Input: part model. Units: mm. Frame: model coordinates. A direction names the side the tool comes from. Give positions to 0.01 mm unless a question says otherwise; leave off trailing zeros. Order: outer loops, then holes, each group sorted by start corner. A loop starts at its lowest first (then second) coordinate and runs counter-clockwise, first axis right, second up.
```python
from build123d import *

# Parameters (mm, degrees)
BOSS_EXTRUDE1_DEPTH                 = 3.175
SKETCH2_R                           = 1.7145
SKETCH2_W                           = 20.586
SKETCH2_H                           = 41.275
CUT_FOR_MOTOR_DEPTH                 = 4.175
SKETCH3_R                           = 3.048
CUT_FOR_AXLE_DEPTH                  = 4.175
SKETCH4_W                           = 6.35
SKETCH4_H                           = 3.2258
CUT_FOR_TABS_DEPTH                  = 4.175
CUT_EXTRUDE6_DEPTH                  = 4.175
SKETCH9_W                           = 3.2258
SKETCH9_H                           = 6.35
TABS_FOR_BACK_PLATE_DEPTH           = 3.175
SKETCH10_R                          = 1.5875
CUT_FOR_BASIC_TILT_LOCK_SCREW_DEPTH = 4.175


with BuildPart() as part:
    # Sketch1 → Boss-Extrude1 (new body)
    with BuildSketch(Plane(origin=(0, 0, 0), x_dir=(0, 0, -1), z_dir=(1, 0, 0))):
        with BuildLine():
            Line((-8.901335672, 27.917328656), (29.198664328, 27.917328656))
            Line((29.198664328, 27.917328656), (52.058664328, 27.917328656))
            ThreePointArc((52.058664328, 27.917328656), (54.100437174, 20.297328656), (52.058664328, 12.677328656))
            Line((52.058664328, 12.677328656), (29.198664328, -0.520898498))
            Line((29.198664328, -0.520898498), (29.198664328, -54.632671344))
            Line((29.198664328, -54.632671344), (-8.901335672, -54.632671344))
            Line((-8.901335672, -54.632671344), (-8.901335672, 27.917328656))
        make_face()
    extrude(amount=BOSS_EXTRUDE1_DEPTH)

    # Sketch2 → cut for motor (cut, through all)
    with BuildSketch(Plane(origin=(3.175, 0, 0), x_dir=(0, 0, -1), z_dir=(1, 0, 0))):
        with Locations((12.696664328, 13.439328656)):
            Circle(SKETCH2_R)
        with Locations((2.786664328, 13.439328656)):
            Circle(SKETCH2_R)
        with Locations((12.595457687, -37.487671344)):
            Circle(SKETCH2_R)
        with Locations((2.685457687, -37.487671344)):
            Circle(SKETCH2_R)
        with Locations((7.741664328, -12.024171344)):
            Rectangle(SKETCH2_W, SKETCH2_H)
    extrude(amount=-CUT_FOR_MOTOR_DEPTH, mode=Mode.SUBTRACT)

    # Sketch3 → cut for axle (cut, through all)
    with BuildSketch(Plane(origin=(3.175, 0, 0), x_dir=(0, 0, -1), z_dir=(1, 0, 0))):
        with Locations((46.978664328, 20.297328656)):
            Circle(SKETCH3_R)
    extrude(amount=-CUT_FOR_AXLE_DEPTH, mode=Mode.SUBTRACT)

    # Sketch4 → cut for tabs (cut, through all)
    with BuildSketch(Plane(origin=(3.175, 0, 0), x_dir=(0, 0, -1), z_dir=(1, 0, 0))):
        with Locations((0.623664328, -49.920971344)):
            Rectangle(SKETCH4_W, SKETCH4_H)
        with Locations((19.673664328, -49.920971344)):
            Rectangle(SKETCH4_W, SKETCH4_H)
        Polygon((10.148664328, -54.632671344), (13.323664328, -54.632671344), (13.323664328, -51.457671344), (6.973664328, -51.457671344), (6.973664328, -54.632671344), align=None)
    extrude(amount=-CUT_FOR_TABS_DEPTH, mode=Mode.SUBTRACT)

    # Sketch8 → Cut-Extrude6 (cut, through all)
    with BuildSketch(Plane(origin=(3.175, 0, 0), x_dir=(0, 0, -1), z_dir=(1, 0, 0))):
        Polygon((29.198664328, 27.917328656), (-8.901335672, 15.979328656), (-8.901335672, 27.917328656), align=None)
    extrude(amount=-CUT_EXTRUDE6_DEPTH, mode=Mode.SUBTRACT)

    # Sketch9 → tabs for back plate (add)
    with BuildSketch(Plane(origin=(3.175, 0, 0), x_dir=(0, 0, -1), z_dir=(1, 0, 0))):
        with Locations((-10.514235672, -6.245671344)):
            Rectangle(SKETCH9_W, SKETCH9_H)
        with Locations((-10.514235672, -18.945671344)):
            Rectangle(SKETCH9_W, SKETCH9_H)
    extrude(amount=-TABS_FOR_BACK_PLATE_DEPTH)

    # Sketch10 → cut for basic tilt lock screw (cut, through all)
    with BuildSketch(Plane(origin=(3.175, 0, 0), x_dir=(0, 0, -1), z_dir=(1, 0, 0))):
        with Locations((36.818664328, 13.947328656)):
            Circle(SKETCH10_R)
    extrude(amount=-CUT_FOR_BASIC_TILT_LOCK_SCREW_DEPTH, mode=Mode.SUBTRACT)


solid = part.part
```
1) Cut plane D-D (x = 2.4). Count the separate pieces of the cut face and the enclosed holes in it, then the cut area to 3 significant figures.
2) First-contact query: P1, Ø1.6, axis at x = 2, y = -53, coming from the +Z side; P2, Ø1.6, axis at x = 2.5, z = -18.5, coming from the +Y side; P3, Ø1.6, axis at x = 1, z = 10, coming from the -Y side; P4, Ø2.5, axis at y = -37.49, z = -2.69, coming from the +X side. Flat tips, straight axial feed; report the tip coordinate or a pass-through.
3) Reachability of faces 1 (the face through (2, -53, -6.974)), 2 (the face through (2, -3.071, 11)), 3 (the face through (2, -13, 8.901)), 4 (the face through (2, -39, 8.901)) from +Z, -Z, +X, -X, +Y, -Y: full face, straight path, thin tool, end or side. Return the list, or none.
4) Cut plane C-C (z = -31.5). Return the cut outline in (x, y) (3 decimals), then the cut area to 3 significant figures.
5) Line query: probe 1 along Y at (x, z) = (1, -2); probe 2 along Z at (x, y) = (1, -37); probe 3 along Z at (x, y) = (0.3, -20.5). Output: solid intervals per line, ascending.
6) Cut plane A-A (y = -11). Return the cut outline in (x, z) (3 decimals), then the cut area to 3 significant figures.
7) Pull-direction query (Y, two-part tool) for faces 5 (the face through (2, -12, -18.035)), 6 (the face through (3.175, -13, -21)), 7 (the face through (1.61, 21.213, -49.886)), 8 (the face through (2, -22.121, 11)); classes: pulls with the +Y half, pulls with the -Y half, needs draft (parallel to the pull), parting line crosses it, or undercut.
8) Cut plane B-B (z = -9.5). Return the cut outline in (x, y) (3 decimals), then the cut area to 3 significant figures.
Geometry says:
1. separate pieces: 1
1. enclosed holes: 9
1. area: 2,490 mm2
2. P1: stops at z = 8.9
2. P2: stops at y = 24.82
2. P3: stops at y = -22.12
2. P4: passes through
3. face 1: +X, -X, -Y
3. face 2: +Z, +X, -X, +Y
3. face 3: +Z, +X, -X
3. face 4: +Z, +X, -X, -Y
4. outline: (0, 0.808) - (3.175, 0.808) - (3.175, 27.917) - (0, 27.917) - close
4. area: 86.1 mm2
5. probe 1: y = -54.63 to -51.53, -48.31 to -39.06, -35.92 to -32.66, 8.61 to 11.92, 14.96 to 19.4
5. probe 2: z = -29.2 to -14.24, -10.95 to -4.33, -1.04 to 8.9
5. probe 3: z = -29.2 to -18.03, 2.55 to 12.13
6. outline: (0, -29.199) - (3.175, -29.199) - (3.175, -18.035) - (0, -18.035) - close; (0, 2.551) - (3.175, 2.551) - (3.175, 8.901) - (0, 8.901) - close
6. area: 55.6 mm2
7. face 5: undercut
7. face 6: needs draft
7. face 7: undercut
7. face 8: pulls with the -Y half
8. outline: (0, -51.458) - (3.175, -51.458) - (3.175, -32.662) - (0, -32.662) - close; (0, 8.613) - (3.175, 8.613) - (3.175, 21.745) - (0, 21.745) - close
8. area: 101 mm2
